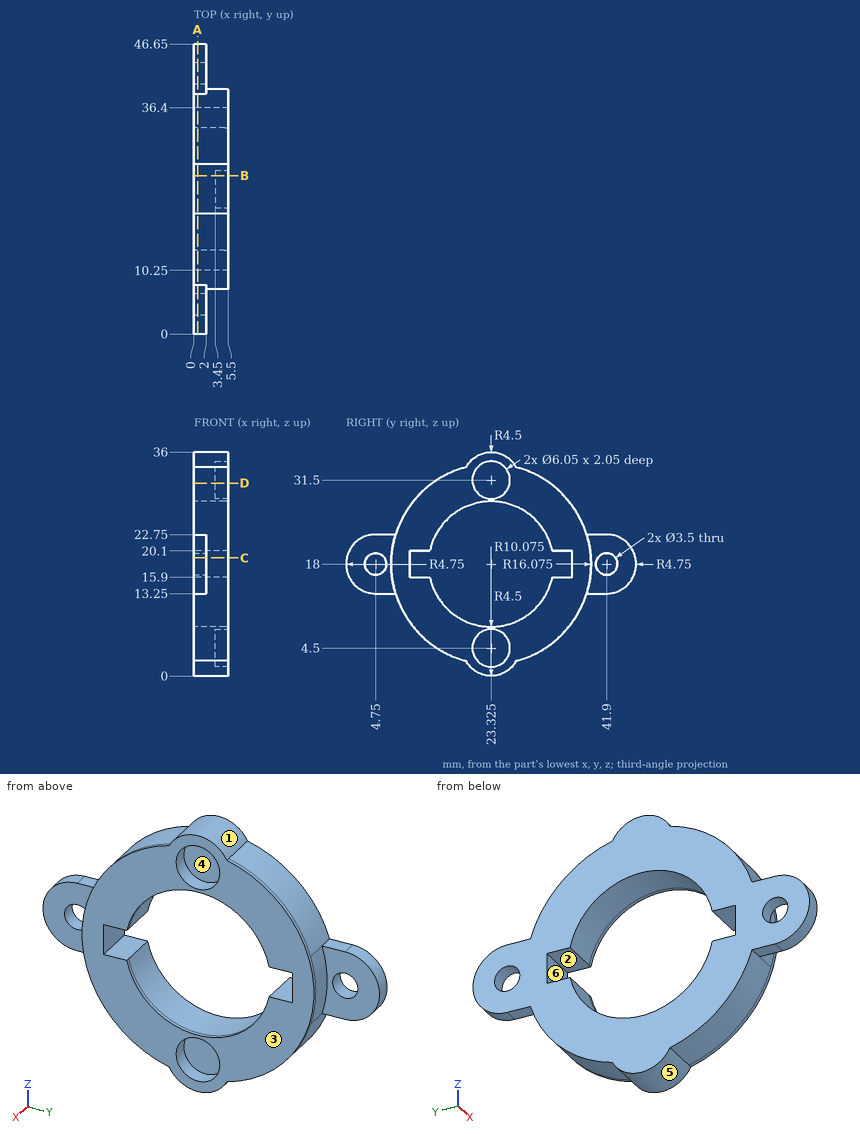
For this review, use the dimensioned drawing (mm, ordinates from the lowest corner) and the shaded views. A direction names the side the tool comes from. Give positions to 0.01 mm unless a question says otherwise; leave off trailing zeros. Order: outer loops, then holes, each group sorted by start corner. A loop starts at its lowest first (then second) coordinate and runs counter-clockwise, first axis right, second up.
1) The part is to be moulded in two halves that separate along Z. For the marked faces 1, 2 and 3, say which applies: released by +Z, released by -Z, zero draft, split by the parting line, or undercut.
2) Insertion check: pin 1 (1.6 mm diameter, centred on x = 3.5, y = 35, fed in from -Z); pin 2 (1.6 mm diameter, centred on x = 1, y = 40, fed in from +Z); pin 3 (5 mm diameter, centred on y = 23.325, z = 31.5, fed in from +X); pin 4 (9 mm diameter, centred on y = 42.5, z = 16, fed in from +X). Each pin has a flat end and moves straight along its axis. Give the tip position at first contact, or say it passes through.
3) Take a section at A-A (x = 0.6). Give the boundary of the cut face in (y, z) (3 decimals), then the cut area to 3 significant figures.
4) For the marked faces 4, 5 and 6, list the 3-axis set-ups (+Z, -Z, +X, -X, +Y, -Y) from which the entire face can be reached by the end or side of a thin tool; tool diameter is ignored.
5) Take a section at B-B (y = 25.5). Give the boundary of the cut face in (x, z).
6) Take a section at D-D (z = 31). Give the boundary of the cut face in (x, y), then the cut area to 3 significant figures.
7) Take a section at C-C (z = 19). Give the boundary of the cut face in (x, y).
8) Wall thickness on line 1 (Y direction, x = 1.25, z = 18); line 2 (Z direction, x = 1.25, y = 4.75); line 3 (Z direction, x = 4.75, y = 24): over which ranges is each line inside the solid? List them lowest first.
Derived:
1. face 1: released by +Z
1. face 2: undercut
1. face 3: zero draft
2. pin 1: stops at z = 6.16
2. pin 2: stops at z = 22.75
2. pin 3: stops at x = 3.45
2. pin 4: stops at x = 5.5
3. outline: (4.75, 13.25) - (7.968, 13.25) arc R16.075 ccw to (19.33, 2.429) arc R4.5 ccw to (27.32, 2.429) arc R16.075 ccw to (38.682, 13.25) - (41.9, 13.25) arc R4.75 ccw to (41.9, 22.75) - (38.682, 22.75) arc R16.075 ccw to (27.32, 33.571) arc R4.5 ccw to (19.33, 33.571) arc R16.075 ccw to (7.968, 22.75) - (4.75, 22.75) arc R4.75 ccw to start; hole circle Ø3.5 at (4.75, 18); hole (10.25, 15.9) - (13.471, 15.9) arc R10.075 ccw to (33.179, 15.9) - (36.4, 15.9) - (36.4, 20.1) - (33.179, 20.1) arc R10.075 ccw to (13.471, 20.1) - (10.25, 20.1) - close; hole circle Ø3.5 at (41.9, 18)
3. area: 593 mm2
4. face 4: +X
4. face 5: -Z, +X, -X
4. face 6: +X, -X
5. outline: (0, 0.56) - (5.5, 0.56) - (5.5, 2.4) - (3.45, 2.4) - (3.45, 6.6) - (5.5, 6.6) - (5.5, 8.16) - (0, 8.16) - close; (0, 27.84) - (5.5, 27.84) - (5.5, 29.4) - (3.45, 29.4) - (3.45, 33.6) - (5.5, 33.6) - (5.5, 35.44) - (0, 35.44) - close
6. outline: (0, 13.87) - (5.5, 13.87) - (5.5, 20.34) - (3.45, 20.34) - (3.45, 26.31) - (5.5, 26.31) - (5.5, 32.78) - (0, 32.78) - close
6. area: 91.8 mm2
7. outline: (0, 0.11) - (2, 0.11) - (2, 3.31) - (0, 3.31) - close; (0, 6.19) - (2, 6.19) - (2, 7.28) - (5.5, 7.28) - (5.5, 10.25) - (0, 10.25) - close; (0, 36.4) - (5.5, 36.4) - (5.5, 39.37) - (2, 39.37) - (2, 40.46) - (0, 40.46) - close; (0, 43.34) - (2, 43.34) - (2, 46.54) - (0, 46.54) - close
8. line 1: y = 0 to 3, 6.5 to 10.25, 36.4 to 40.15, 43.65 to 46.65
8. line 2: z = 13.25 to 16.25, 19.75 to 22.75
8. line 3: z = 0.05 to 1.55, 7.45 to 7.95, 28.05 to 28.55, 34.45 to 35.95
